Model file for the job. Use its own axes, mm. A direction names the side the tool comes from. Coordinates: 2 decimals unless noted, no trailing zeros. Write each loop counter-clockwise with the first axis right and the second up, starting at its lowest first coordinate (ties: lowest second). Pieces come first, ordered by that corner, then holes. Notation, with made-up numbers: M -15,-6.75 L 31,-6.75 A24 cw 31,14.25 Z; hole C 9,-15 d8. An arc over 180 degrees is marked long. Answer in a Markdown table with one row per item. Add a question column.
```python
from build123d import *

# Parameters (mm, degrees)
SKETCH1_R               = 4.825
SKETCH1_R_2             = 1.818202682
BOSS_EXTRUDE1_DEPTH     = 15
SKETCH2_W               = 15
SKETCH2_H               = 10
BOSS_EXTRUDE2_DEPTH     = 5
SKETCH3_W               = 0.5
SKETCH3_H               = 1.5
BOSS_EXTRUDE3_DEPTH     = 3
SKETCH4_W               = 0.5
SKETCH4_H               = 1.5
BOSS_EXTRUDE4_DEPTH     = 10
LPATTERN2_COUNT         = 4
LPATTERN2_PITCH         = 2.5
MIRROR1_COPY_1_SKETCH_W = 0.5
MIRROR1_COPY_1_SKETCH_H = 1.5
MIRROR1_COPY_1_DEPTH    = 3
MIRROR1_COPY_2_SKETCH_W = 0.5
MIRROR1_COPY_2_SKETCH_H = 1.5
MIRROR1_COPY_2_DEPTH    = 3
MIRROR1_COPY_3_SKETCH_W = 0.5
MIRROR1_COPY_3_SKETCH_H = 1.5
MIRROR1_COPY_3_DEPTH    = 3
MIRROR1_COPY_4_SKETCH_W = 0.5
MIRROR1_COPY_4_SKETCH_H = 1.5
MIRROR1_COPY_4_DEPTH    = 10
MIRROR1_COPY_5_SKETCH_W = 0.5
MIRROR1_COPY_5_SKETCH_H = 1.5
MIRROR1_COPY_5_DEPTH    = 10
MIRROR1_COPY_6_SKETCH_W = 0.5
MIRROR1_COPY_6_SKETCH_H = 1.5
MIRROR1_COPY_6_DEPTH    = 10


with BuildPart() as part:
    # Sketch1 → Boss-Extrude1 (new body)
    with BuildSketch(Plane.XY):
        Circle(SKETCH1_R)
        Circle(SKETCH1_R_2, mode=Mode.SUBTRACT)
    extrude(amount=BOSS_EXTRUDE1_DEPTH)

    # Sketch2 → Boss-Extrude2 (add)
    with BuildSketch(Plane.XY.offset(15)):
        Rectangle(SKETCH2_W, SKETCH2_H)
    extrude(amount=BOSS_EXTRUDE2_DEPTH)

    # Sketch3 → Boss-Extrude3 (add)
    with BuildSketch(Plane.ZY.offset(7.5)):
        with Locations((19.330067801, 3.591756208)):
            Rectangle(SKETCH3_W, SKETCH3_H)
    boss_extrude3 = extrude(amount=BOSS_EXTRUDE3_DEPTH)

    # Sketch4 → Boss-Extrude4 (add)
    with BuildSketch(Plane.XY.offset(19.580067801)):
        with Locations((-10.25, 3.591756208)):
            Rectangle(SKETCH4_W, SKETCH4_H)
    boss_extrude4 = extrude(amount=BOSS_EXTRUDE4_DEPTH)

    # LPattern2: Boss-Extrude3, Boss-Extrude4 ×4
    with Locations(*[(0, -i * LPATTERN2_PITCH, 0) for i in range(1, LPATTERN2_COUNT)]):
        add(boss_extrude3)
        add(boss_extrude4)

    # Mirror1: Boss-Extrude3, Boss-Extrude4 across plane
    add(boss_extrude3.mirror(Plane(origin=(0, 0, 0), x_dir=(0, 0, 1), z_dir=(1, 0, 0))))
    add(boss_extrude4.mirror(Plane(origin=(0, 0, 0), x_dir=(0, 0, 1), z_dir=(1, 0, 0))))

    # Mirror1 copy 1 sketch → Mirror1 copy 1 (add)
    with BuildSketch(Plane(origin=(7.5, -2.5, 0), x_dir=(0, 0, 1), z_dir=(1, 0, 0))):
        with Locations((19.330067801, -3.591756208)):
            Rectangle(MIRROR1_COPY_1_SKETCH_W, MIRROR1_COPY_1_SKETCH_H)
    extrude(amount=MIRROR1_COPY_1_DEPTH)

    # Mirror1 copy 2 sketch → Mirror1 copy 2 (add)
    with BuildSketch(Plane(origin=(7.5, -5, 0), x_dir=(0, 0, 1), z_dir=(1, 0, 0))):
        with Locations((19.330067801, -3.591756208)):
            Rectangle(MIRROR1_COPY_2_SKETCH_W, MIRROR1_COPY_2_SKETCH_H)
    extrude(amount=MIRROR1_COPY_2_DEPTH)

    # Mirror1 copy 3 sketch → Mirror1 copy 3 (add)
    with BuildSketch(Plane(origin=(7.5, -7.5, 0), x_dir=(0, 0, 1), z_dir=(1, 0, 0))):
        with Locations((19.330067801, -3.591756208)):
            Rectangle(MIRROR1_COPY_3_SKETCH_W, MIRROR1_COPY_3_SKETCH_H)
    extrude(amount=MIRROR1_COPY_3_DEPTH)

    # Mirror1 copy 4 sketch → Mirror1 copy 4 (add)
    with BuildSketch(Plane(origin=(0, -2.5, 19.580067801), x_dir=(-1, 0, 0), z_dir=(0, 0, 1))):
        with Locations((-10.25, -3.591756208)):
            Rectangle(MIRROR1_COPY_4_SKETCH_W, MIRROR1_COPY_4_SKETCH_H)
    extrude(amount=MIRROR1_COPY_4_DEPTH)

    # Mirror1 copy 5 sketch → Mirror1 copy 5 (add)
    with BuildSketch(Plane(origin=(0, -5, 19.580067801), x_dir=(-1, 0, 0), z_dir=(0, 0, 1))):
        with Locations((-10.25, -3.591756208)):
            Rectangle(MIRROR1_COPY_5_SKETCH_W, MIRROR1_COPY_5_SKETCH_H)
    extrude(amount=MIRROR1_COPY_5_DEPTH)

    # Mirror1 copy 6 sketch → Mirror1 copy 6 (add)
    with BuildSketch(Plane(origin=(0, -7.5, 19.580067801), x_dir=(-1, 0, 0), z_dir=(0, 0, 1))):
        with Locations((-10.25, -3.591756208)):
            Rectangle(MIRROR1_COPY_6_SKETCH_W, MIRROR1_COPY_6_SKETCH_H)
    extrude(amount=MIRROR1_COPY_6_DEPTH)


solid = part.part
```
1) Two-plate mould, pull along X, no slides. Class faces 1 (the face through (9, 4, 19.58)), 2 (the face through (-5, 0, 15)), 3 (the face through (-10.5, -4, 24)): released by +X, released by -X, zero draft, split by the parting line, or undercut.
2) Flat gauge pins, fed straight in: pin 1 Ø0.5 at (x, y) = (-8.5, -4) entering from +Z; pin 2 Ø1.5 at (x, z) = (-9.5, 25) entering from +Y; pin 3 Ø1.5 at (x, y) = (-6, -2.5) entering from -Z; pin 4 Ø6 at (x, y) = (0.5, 3) entering from -Z. Where does each tip first touch, or does it go through?
3) Drill centre lines: probe 1 along Y at (x, z) = (0, 11) (3 decimals); probe 2 along Z at (x, y) = (-5.25, -4); probe 3 along Z at (x, y) = (-4.5, 1.25). Where is each one in solid material? Low to high.
4) Slice it at D-D (x = 0). Give the cut face in (y, z) (3 decimals), then the cut area to 3 significant figures.
5) Which spindle directions (+Z, -Z, +X, -X, +Y, -Y) get a long thin tool onto all of the face, cutting with end or side? Do faces 4 (the face through (9, -4, 19.08)), 5 (the face through (10.3, -4.658, 23.5)), 6 (the face through (-9, -4, 19.58)), 7 (the face through (-9, -4, 19.08)). Say none if no direction does.
6) Slice it at B-B (z = 22.5). Count the separate pieces of the cut face and the enclosed holes in it, then the cut area to 3 significant figures.
7) Slice it at C-C (y = 0). Give the cut face in (x, z) (3 decimals), then the cut area to 3 significant figures.
8) Slice it at A-A (x = 8.25). Give the cut face in (y, z).
Ans:
| question | item | result |
|---|---|---|
| 1 | face 1 | undercut |
| 1 | face 2 | zero draft |
| 1 | face 3 | released by -X |
| 2 | pin 1 | stops at z = 19.58 |
| 2 | pin 2 | stops at y = 4.34 |
| 2 | pin 3 | stops at z = 15 |
| 2 | pin 4 | stops at z = 0 |
| 3 | probe 1 | y = -4.825 to -1.818, 1.818 to 4.825 |
| 3 | probe 2 | z = 15 to 20 |
| 3 | probe 3 | z = 0 to 20 |
| 4 | outline | M -5,15 L -4.825,15 L -4.825,0 L -1.818,0 L -1.818,15 L 1.818,15 L 1.818,0 L 4.825,0 L 4.825,15 L 5,15 L 5,20 L -5,20 Z |
| 4 | area | 140 mm2 |
| 5 | face 4 | -Z, +X, +Y, -Y |
| 5 | face 5 | +Z, -Z, +X, -Y |
| 5 | face 6 | +Z, +Y, -Y |
| 5 | face 7 | -Z, -X, +Y, -Y |
| 6 | separate pieces | 8 |
| 6 | enclosed holes | 0 |
| 6 | area | 6.00 mm2 |
| 7 | outline | M -7.5,15 L -4.825,15 L -4.825,0 L -1.818,0 L -1.818,15 L 1.818,15 L 1.818,0 L 4.825,0 L 4.825,15 L 7.5,15 L 7.5,20 L -7.5,20 Z |
| 7 | area | 165 mm2 |
| 8 | outline | M -4.66,19.08 L -3.16,19.08 L -3.16,19.58 L -4.66,19.58 Z; M -2.16,19.08 L -0.66,19.08 L -0.66,19.58 L -2.16,19.58 Z; M 0.34,19.08 L 1.84,19.08 L 1.84,19.58 L 0.34,19.58 Z; M 2.84,19.08 L 4.34,19.08 L 4.34,19.58 L 2.84,19.58 Z |
